Here's the drawing with two shaded views (mm, measured from the low corner). I have some questions. Round coordinates to 2 decimals unless told otherwise and drop trailing zeros. Order: outer loops, then holes, each group sorted by start corner. A loop starts at its lowest first (then second) coordinate and runs counter-clockwise, first axis right, second up. Notation, with made-up numbers: (48, 30) - (104, 30) arc R30 cw to (104, 67) - close; hole circle Ø10 at (19, 24.25). An arc over 180 degrees is marked (long way). One line per item, written item: value.
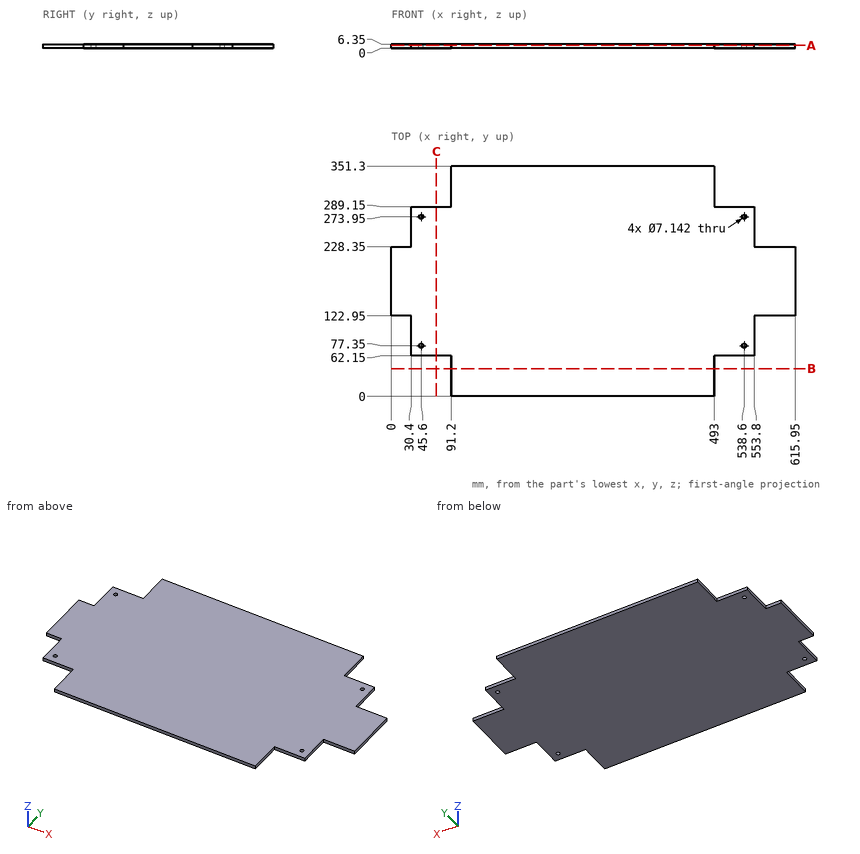
Q1. If I drill on line 1 along Y through (x, z) = (45.6, 4.25); line 2 along X through (y, z) = (273.95, 1.5); line 3 along X through (y, z) = (121.5, 5.25), over which ranges is the centre line in solid material (lowest first)?
Results list:
line 1: 62.15 to 73.78, 80.92 to 270.38, 277.52 to 289.15
line 2: 30.4 to 42.03, 49.17 to 535.03, 542.17 to 553.8
line 3: 30.4 to 553.8
Q2. If we section it at A-A, the plane z = 4.25: Please give me the cut outline in (x, y).
Results list:
outline: (0, 122.95) - (30.4, 122.95) - (30.4, 62.15) - (91.2, 62.15) - (91.2, 0) - (493, 0) - (493, 62.15) - (553.8, 62.15) - (553.8, 122.95) - (615.95, 122.95) - (615.95, 228.35) - (553.8, 228.35) - (553.8, 289.15) - (493, 289.15) - (493, 351.3) - (91.2, 351.3) - (91.2, 289.15) - (30.4, 289.15) - (30.4, 228.35) - (0, 228.35) - close; hole circle Ø7.14 at (45.6, 77.35); hole circle Ø7.14 at (45.6, 273.95); hole circle Ø7.14 at (538.6, 77.35); hole circle Ø7.14 at (538.6, 273.95)
Q3. Will these pins go through, and if not, where does the flat tip stop? pin 1 (4.5 mm diameter, centred on x = 45.6, y = 273.95, fed in from -Z); pin 2 (1.9 mm diameter, centred on x = 576.5, z = 2, fed in from -Y); pin 3 (2 mm diameter, centred on y = 115, z = 4, fed in from -X); pin 4 (1.9 mm diameter, centred on x = 583, z = 4, fed in from +Y).
Results list:
pin 1: through
pin 2: y = 122.95
pin 3: x = 30.4
pin 4: y = 228.35
Q4. If we section it at B-B, the plane y = 42.5: Please give me the cut outline in (x, z), then the cut area to 3 significant figures.
Results list:
outline: (91.2, 0) - (493, 0) - (493, 6.35) - (91.2, 6.35) - close
area: 2,550 mm²
Q5. If we section it at C-C, the plane x = 69: Please give me the cut outline in (y, z).
Results list:
outline: (62.15, 0) - (289.15, 0) - (289.15, 6.35) - (62.15, 6.35) - close
